Read the model definition and answer for the solid it produces. Units are mm, in the model's axes. Coordinates: 2 decimals unless noted, no trailing zeros. Loops run counter-clockwise (first coordinate to the right, second up) from the corner with the lowest first, then second, coordinate; pieces in that order, holes last. Notation, with made-up numbers: M 29,41 L 72,41 A18 ccw 72,50 Z; hole C -22.75,11.25 d7. An arc over 180 degrees is marked long. Put each result on its own line as item: value.
from build123d import *

# Parameters (mm, degrees)
SKETCH1_R           = 150
BOSS_EXTRUDE1_DEPTH = 100
FILLET1_R           = 20
SKETCH2_R           = 40
CUT_EXTRUDE1_DEPTH  = 101


with BuildPart() as part:
    # Sketch1 → Boss-Extrude1 (new body)
    with BuildSketch(Plane(origin=(0, 0, 0), x_dir=(0, 0, -1), z_dir=(1, 0, 0))):
        Circle(SKETCH1_R)
    extrude(amount=BOSS_EXTRUDE1_DEPTH)

    # Fillet1
    fillet1_edges = [part.edges().sort_by_distance(p)[0] for p in [
        (0, 0, 150),
        (100, 0, 150),
    ]]
    fillet(fillet1_edges, radius=FILLET1_R)

    # Sketch2 → Cut-Extrude1 (cut, through all)
    with BuildSketch(Plane.ZY):
        Circle(SKETCH2_R)
    extrude(amount=-CUT_EXTRUDE1_DEPTH, mode=Mode.SUBTRACT)


solid = part.part
1) Straight lines are drawn through the part: line 1 (Y direction, x = 45, z = 0); line 2 (Z direction, x = 57.5, y = 34.5); line 3 (Z direction, x = 50.5, y = 37). For each, find the intervals that lie inside material, in ascending order. Write a range as [from, to].
Answer list:
line 1: y = [-150, -40], [40, 150]
line 2: z = [-145.98, -20.24], [20.24, 145.98]
line 3: z = [-145.37, -15.2], [15.2, 145.37]
2) Find section A-A, the plane z = 0. Write down the section's boundary in (x, y), plus the area to 3 significant figures.
Answer list:
outline: M 0,-130 A20 ccw 20,-150 L 80,-150 A20 ccw 100,-130 L 100,-40 L 0,-40 Z; M 0,40 L 100,40 L 100,130 A20 ccw 80,150 L 20,150 A20 ccw 0,130 Z
area: 21,700 mm^2
3) Given pin 1 Ø5 at (x, y) = (16, 4) entering from +Z; pin 2 Ø8 at (x, z) = (19.5, -101.5) entering from +Y; pin 3 Ø1.5 at (x, y) = (61, 88) entering from -Z; pin 4 Ø3 at (y, z) = (-36.5, 40.5) entering from -X, each flat-ended and moving along its own axis, determine where each tip first touches the part or whether it passes through.
Answer list:
pin 1: stops at z = 149.9
pin 2: stops at y = 113.98
pin 3: stops at z = -122.01
pin 4: stops at x = 0
4) Find section C-C, the plane x = 47.5. Write down the section's boundary in (y, z), plus the area to 3 significant figures.
Answer list:
outline: C 0,0 d300; hole C 0,0 d80
area: 65,700 mm^2
5) Determine the mould class of faces 1 (the flat face through (0, 31, -27)), 2 (the cylindrical face through (49.3, -39.05, -8.67)), 3 (the cylindrical face through (49.58, 148.724, 19.527)) for opening direction Z: released by +Z, released by -Z, zero draft, split by the parting line, or undercut.
Answer list:
face 1: zero draft
face 2: undercut
face 3: split by the parting line
